```python
from build123d import *

# Parameters (mm, degrees)
SKETCH1_W               = 45.5
SKETCH1_H               = 37
SKETCH1_W_2             = 10.66
SKETCH1_H_2             = 4
BOSS_EXTRUDE1_DEPTH     = 4
SKETCH3_R               = 1.6
CUT_EXTRUDE5_DEPTH      = 10
CUT_EXTRUDE5_DEPTH_BACK = 1
SKETCH4_R               = 2.35
LEGO_GATEN_DEPTH        = 10


with BuildPart() as part:
    # Sketch1 → Boss-Extrude1 (new body)
    with BuildSketch(Plane.XY):
        with Locations((22.75, 18.5)):
            Rectangle(SKETCH1_W, SKETCH1_H)
        with Locations((22.75, 32.14)):
            Rectangle(SKETCH1_W_2, SKETCH1_H_2, mode=Mode.SUBTRACT)
    extrude(amount=BOSS_EXTRUDE1_DEPTH)

    # Sketch3 → Cut-Extrude5 (cut, two sides)
    with BuildSketch(Plane.XY) as cut_extrude5_sk:
        with Locations((41.27584891, 32.252592082)):
            Circle(SKETCH3_R)
        with Locations((41.27584891, 12.252592082)):
            Circle(SKETCH3_R)
        with Locations((4.27584891, 12.252592082)):
            Circle(SKETCH3_R)
        with Locations((4.27584891, 32.252592082)):
            Circle(SKETCH3_R)
    extrude(amount=CUT_EXTRUDE5_DEPTH, mode=Mode.SUBTRACT)
    extrude(cut_extrude5_sk.sketch, amount=-CUT_EXTRUDE5_DEPTH_BACK, mode=Mode.SUBTRACT)

    # Sketch4 → Lego gaten (cut)
    with BuildSketch(Plane.XY.offset(4)):
        with Locations((10.78, 8)):
            Circle(SKETCH4_R)
        with Locations((18.76, 8)):
            Circle(SKETCH4_R)
        with Locations((26.74, 8)):
            Circle(SKETCH4_R)
        with Locations((34.72, 8)):
            Circle(SKETCH4_R)
    extrude(amount=-LEGO_GATEN_DEPTH, mode=Mode.SUBTRACT)


solid = part.part
```
Model file for the job. Use its own axes, mm. A direction names the side the tool comes from. Coordinates: 2 decimals unless noted, no trailing zeros. Loops run counter-clockwise (first coordinate to the right, second up) from the corner with the lowest first, then second, coordinate; pieces in that order, holes last. Notation, with made-up numbers: (10.5, -27.75) -> (40.5, -27.75) arc R22 cw to (40.5, 9.25) -> close; hole circle Ø2 at (-33.75, 12.25). An arc over 180 degrees is marked (long way). Answer as a JSON object with one key per item and string values.
Q1. Cut at C-C (x = 18.76). List the corners of the cut face in (y, z), and give its area (3 significant figures).
Report:
{"outline": "(0, 0) -> (5.65, 0) -> (5.65, 4) -> (0, 4) -> close; (10.35, 0) -> (30.14, 0) -> (30.14, 4) -> (10.35, 4) -> close; (34.14, 0) -> (37, 0) -> (37, 4) -> (34.14, 4) -> close", "area": "113 mm2"}
Q2. Pull direction X, two halves, no side cores. Call faces 3 (the flat face through (0, 18, 2)), 4 (the cylindrical face through (4.07, 33.84, 1.97)), 5 (the flat face through (22, 19, 0)): released by +X, released by -X, zero draft, split by the parting line, or undercut.
Report:
{"face 3": "released by -X", "face 4": "undercut", "face 5": "zero draft"}
Q3. Cut at A-A (x = 10.78). List the corners of the cut face in (y, z).
Report:
{"outline": "(0, 0) -> (5.65, 0) -> (5.65, 4) -> (0, 4) -> close; (10.35, 0) -> (37, 0) -> (37, 4) -> (10.35, 4) -> close"}
Q4. 3-axis set-ups, long thin cutter, end or side, ignore diameter. For faces 1 (the flat face through (22, 19, 4)), 2 (the flat face through (23, 34.14, 2)): which of +Z, -Z, +X, -X, +Y, -Y reach the whole face in a straight line?
Report:
{"face 1": "+Z, +X, -X, +Y, -Y", "face 2": "+Z, -Z"}
Q5. Cut at B-B (y = 8). List the corners of the cut face in (x, z).
Report:
{"outline": "(0, 0) -> (8.43, 0) -> (8.43, 4) -> (0, 4) -> close; (13.13, 0) -> (16.41, 0) -> (16.41, 4) -> (13.13, 4) -> close; (21.11, 0) -> (24.39, 0) -> (24.39, 4) -> (21.11, 4) -> close; (29.09, 0) -> (32.37, 0) -> (32.37, 4) -> (29.09, 4) -> close; (37.07, 0) -> (45.5, 0) -> (45.5, 4) -> (37.07, 4) -> close"}
Q6. Cut at D-D (z = 1.5). State how many separate pieces and enclosed holes the cut face has, and give its area (3 significant figures).
Report:
{"separate pieces": "1", "enclosed holes": "9", "area": "1,540 mm2"}
Q7. Probe probe 1 along Y at (x, z) = (26.74, 1.2); probe 2 along X at (y, z) = (11.5, 3.4); probe 3 along Y at (x, z) = (23.5, 3.3). List the from-to ranges inside material, lowest first.
Report:
{"probe 1": "y = 0 to 5.65, 10.35 to 30.14, 34.14 to 37", "probe 2": "x = 0 to 2.86, 5.69 to 39.86, 42.69 to 45.5", "probe 3": "y = 0 to 30.14, 34.14 to 37"}
Q8. Flat gauge pin, fed straight in: P1, Ø3, axis at x = 4.28, y = 12.25, coming from the +Z side. Where does the tip first touch, or does it go through?
Report:
{"P1": "passes through"}
